Could you check a few things on this drawing? It's one solid part, dimensions in mm from its lowest x, y, z. Coordinates: 2 decimals unless noted, no trailing zeros. Loops run counter-clockwise (first coordinate to the right, second up) from the corner with the lowest first, then second, coordinate; pieces in that order, holes last. Notation, with made-up numbers: M 88.25,-5.5 L 146.25,-5.5 A32 ccw 146.25,29.5 Z; hole C 52,52.5 d9. An arc over 180 degrees is marked long. Answer as a JSON object with one key per item and string values. Group by question number.
Item 1: If I drill on line 1 (Z direction, x = 109, y = 0.4); line 2 (X direction, y = 2.25, z = 127) (1 decimal); line 3 (Z direction, x = 158, y = 0.3) (1 decimal), over which ranges is the centre line in solid material (lowest first)?
Item 2: I'm going to push a flat-ended pin straight in: pin 1 Ø1.5 at (y, z) = (2.5, 167.5) entering from -X (1 decimal). Where does the tip first touch, or does it pass through?
Item 3: Suppose I cut it at A-A (y = 1.5). Write out the boundary of the cut face in (x, z), then the cut area to 3 significant figures.
Item 4: Suppose I cut it at B-B (z = 195.5). Write out the boundary of the cut face in (x, y), then the cut area to 3 significant figures.
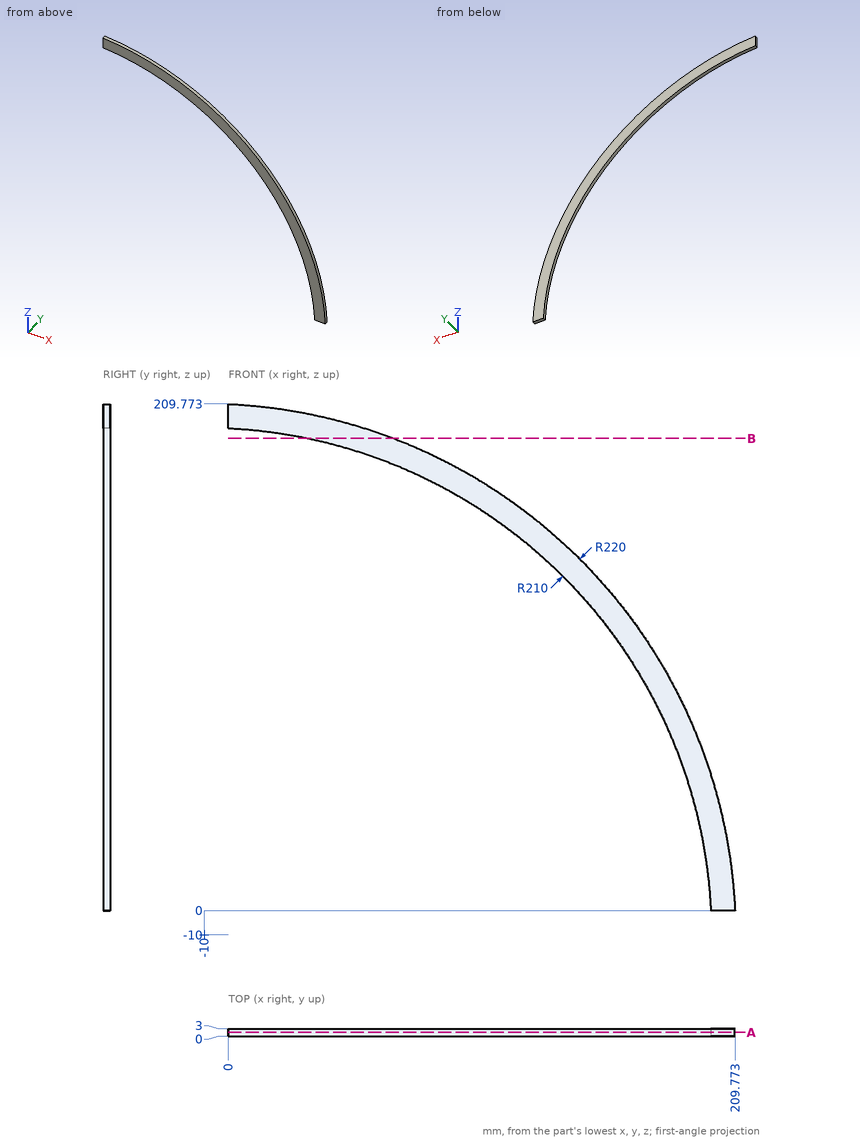
From the geometry:
{
 "1": {"line 1": "163.03 to 175.04", "line 2": "149.2 to 162.1", "line 3": "116 to 132"},
 "2": {"pin 1": "x = 101"},
 "3": {"outline": "M 0,199.76 A210 cw 199.76,0 L 209.77,0 A220 ccw 0,209.77 Z", "area": "3,180 mm2"},
 "4": {"outline": "M 33.24,0 L 68.55,0 L 68.55,3 L 33.24,3 Z", "area": "106 mm2"}
}
